Check sheet for the modelled part. Datum: model origin and axes. Units: mm. Coordinates: 2 decimals unless noted, no trailing zeros. Loops run counter-clockwise (first coordinate to the right, second up) from the corner with the lowest first, then second, coordinate; pieces in that order, holes last. Notation, with made-up numbers: (25, 22.5) - (69, 22.5) arc R18 ccw to (69, 50.5) - close; hole circle Ø7 at (63.5, 80.25). An arc over 180 degrees is marked (long way). Write each question's results on one line, items separated by ' | '. Start each with the question number.
1. Cross-section at C-C (x = -32). Record the cut outline in (y, z).
2. Thickness scan on line 1 (X direction, y = -1.25, z = -17.5); line 2 (X direction, y = -15, z = 19); line 3 (Z direction, x = 6, y = -3.5). Record the ranges inside material, lowest first. Write a range as [from, to].
3. Cross-section at A-A (z = 23.5). Record the cut outline in (x, y), and give its area (3 significant figures).
4. Cross-section at B-B (y = -12.5). Record the cut outline in (x, z) (3 decimals).
5. Cross-section at D-D (z = -26.5). Record the cut outline in (x, y).
6. Gauge pin test, flat ends, axial feed: P1, Ø8, axis at y = -5.5, z = -52, coming from the -X side; P2, Ø6, axis at y = -9, z = -37.5, coming from the -X side; P3, Ø12, axis at x = -36.5, z = -33.5, coming from the +Y side; P4, Ø2, axis at y = -14.5, z = -19, coming from the -X side. Record the tip position at first contact, or that the pin passes through.
```python
from build123d import *

# Parameters (mm, degrees)
F1_DEPTH = 25.4


with BuildPart() as f1:
    # F0 (on Front) → F1 (new body)
    with BuildSketch(Plane.XZ):
        with BuildLine():
            ThreePointArc((-55.88, 71.755), (-45.7062069243, 69.2896700239), (-37.7894898478, 62.4406183985))
            Line((-37.7894898478, 62.4406183985), (-40.9707072614, 75.4116006232))
            Line((-40.9707072614, 75.4116006232), (-55.88, 71.755))
        make_face()
        with BuildLine():
            ThreePointArc((20.1514706795, -9.3738388323), (-0.0637628383, -22.224908533), (-20.2049252332, -9.2580571029))
            ThreePointArc((-20.2049252332, -9.2580571029), (-21.5852935507, -5.293933068), (-22.1956935913, -1.1409693254))
            Line((-22.1956935913, -1.1409693254), (-33.8688111264, 46.4545830573))
            ThreePointArc((-33.8688111264, 46.4545830573), (-49.7758218318, 28.1597020636), (-72.9459940838, 35.2926382032))
            Line((-72.9459940838, 35.2926382032), (-50.7529312723, -55.1965631947))
            ThreePointArc((-50.7529312723, -55.1965631947), (-35.536234837, -38.1117715463), (-19.05, -53.975))
            ThreePointArc((-19.05, -53.975), (-22.7428404887, -64.153929936), (-32.1033057816, -69.5972170878))
            Line((-32.1033057816, -69.5972170878), (33.760778806, -69.8072523354))
            ThreePointArc((33.760778806, -69.8072523354), (22.7534984393, -43.7833281666), (50.3064695665, -50.0474029008))
            Line((50.3064695665, -50.0474029008), (73.6114514871, 36.1305129516))
            ThreePointArc((73.6114514871, 36.1305129516), (51.7301219198, 27.695872197), (34.4690239948, 43.5700728609))
            Line((34.4690239948, 43.5700728609), (22.1293157515, -2.0600993596))
            ThreePointArc((22.1293157515, -2.0600993596), (21.4543450512, -5.8018706833), (20.1514706795, -9.3738388323))
        make_face()
        with BuildLine():
            Line((43.1457490814, 75.6551475002), (40.391048509, 65.4687266339))
            ThreePointArc((40.391048509, 65.4687266339), (48.4732019865, 70.4844737034), (57.912088459, 71.6619055098))
            Line((57.912088459, 71.6619055098), (43.1457490814, 75.6551475002))
        make_face()
        with BuildLine():
            Line((40.391048509, 65.4687266339), (34.4690239948, 43.5700728609))
            ThreePointArc((34.4690239948, 43.5700728609), (51.7301219198, 27.695872197), (73.6114514871, 36.1305129516))
            ThreePointArc((73.6114514871, 36.1305129516), (76.9516887589, 42.4635611621), (78.105, 49.53))
            ThreePointArc((78.105, 49.53), (74.6263449007, 61.4683909244), (65.2793372, 69.6695899958))
            Line((65.2793372, 69.6695899958), (57.912088459, 71.6619055098))
            ThreePointArc((57.912088459, 71.6619055098), (48.4732019865, 70.4844737034), (40.391048509, 65.4687266339))
        make_face()
        with BuildLine():
            ThreePointArc((50.8, -53.975), (50.6761341555, -51.9957582726), (50.3064695665, -50.0474029008))
            ThreePointArc((50.3064695665, -50.0474029008), (22.7534984393, -43.7833281666), (33.760778806, -69.8072523354))
            Line((33.760778806, -69.8072523354), (35.988222994, -69.8143554751))
            ThreePointArc((35.988222994, -69.8143554751), (46.5201345406, -64.8178999804), (50.8, -53.975))
        make_face()
        with BuildLine():
            ThreePointArc((-19.05, -53.975), (-35.536234837, -38.1117715463), (-50.7529312723, -55.1965631947))
            ThreePointArc((-50.7529312723, -55.1965631947), (-46.7400785083, -64.577808347), (-37.8462717948, -69.5789032329))
            Line((-37.8462717948, -69.5789032329), (-32.1033057816, -69.5972170878))
            ThreePointArc((-32.1033057816, -69.5972170878), (-22.7428404887, -64.153929936), (-19.05, -53.975))
        make_face()
        with BuildLine():
            ThreePointArc((-72.9459940838, 35.2926382032), (-49.7758218318, 28.1597020636), (-33.8688111264, 46.4545830573))
            Line((-33.8688111264, 46.4545830573), (-37.7894898478, 62.4406183985))
            ThreePointArc((-37.7894898478, 62.4406183985), (-45.7062069243, 69.2896700239), (-55.88, 71.755))
            ThreePointArc((-55.88, 71.755), (-76.0092820405, 58.9513921229), (-72.9459940838, 35.2926382032))
        make_face()
    extrude(amount=F1_DEPTH)


solid = f1.part
```
Established:
1) outline: (-25.4, -69.6) - (0, -69.6) - (0, 38.83) - (-25.4, 38.83) - close
2) line 1: [-60, -13.7], [13.7, 59.11] | line 2: [-68.95, -27.14], [27.82, 68.98] | line 3: [-69.72, -21.4]
3) outline: (-70.05, -25.4) - (-28.24, -25.4) - (-28.24, 0) - (-70.05, 0) - close; (29.04, -25.4) - (70.2, -25.4) - (70.2, 0) - (29.04, 0) - close | area: 2,110 mm^2
4) outline: (-72.946, 35.293) - (-50.753, -55.197) arc R15.875 ccw to (-37.846, -69.579) - (35.988, -69.814) arc R15.875 ccw to (50.306, -50.047) - (73.611, 36.131) arc R22.225 ccw to (65.279, 69.67) - (43.146, 75.655) - (22.129, -2.06) arc R22.225 cw to (-22.196, -1.141) - (-40.971, 75.412) - (-55.88, 71.755) arc R22.225 ccw to start
5) outline: (-57.79, -25.4) - (56.67, -25.4) - (56.67, 0) - (-57.79, 0) - close
6) P1: x = -52.52 | P2: x = -55.83 | P3: y = 0 | P4: x = -59.88
